Build history of the part. All positions in model axes, mm. Round coordinates to 2 decimals unless told otherwise and drop trailing zeros. Order: outer loops, then holes, each group sorted by start corner. A loop starts at its lowest first (then second) coordinate and runs counter-clockwise, first axis right, second up. Notation, with made-up numbers: (13, -22.75) -> (50, -22.75) arc R25 ccw to (50, -6.75) -> close; hole circle Ø4 at (-33, 29.5). An arc over 180 degrees is marked (long way). Answer as a JSON object with one key per item and string values.
from build123d import *

# Parameters (mm, degrees)
SKETCH_W  = 7
SKETCH_H  = 7
PAD_DEPTH = 60


with BuildPart() as part:
    # Sketch → Pad (new body)
    with BuildSketch(Plane.XY):
        Rectangle(SKETCH_W, SKETCH_H)
        with BuildLine():
            ThreePointArc((-1.349854, 1.608693), (0, -2.1), (1.349854, 1.608693))
            Line((0.764337, 2.1), (1.349854, 1.608693))
            Line((-0.764337, 2.1), (0.764337, 2.1))
            Line((-0.764337, 2.1), (-1.349854, 1.608693))
        make_face(mode=Mode.SUBTRACT)
    extrude(amount=PAD_DEPTH)


solid = part.part
1) Cut at A-A, the plane y = 0. Give the cut face in (x, z), plus the area to 3 significant figures.
Checked values:
{"outline": "(-3.5, 0) -> (-2.1, 0) -> (-2.1, 60) -> (-3.5, 60) -> close; (2.1, 0) -> (3.5, 0) -> (3.5, 60) -> (2.1, 60) -> close", "area": "168 mm²"}
2) Probe L1, parallel to Y at x = 0, z = 25; L2, parallel to Y at x = 1.25, z = 57. List the from-to ranges inside material, lowest first. Write a range as from..to.
Checked values:
{"L1": "y = -3.5..-2.1, 2.1..3.5", "L2": "y = -3.5..-1.69, 1.69..3.5"}
3) Cut at B-B, the plane z = 24.5. Give the cut face in (x, y), plus the area to 3 significant figures.
Checked values:
{"outline": "(-3.5, -3.5) -> (3.5, -3.5) -> (3.5, 3.5) -> (-3.5, 3.5) -> close; hole (-1.35, 1.61) arc R2.1 ccw (long way) to (1.35, 1.61) -> (0.76, 2.1) -> (-0.76, 2.1) -> close", "area": "35.0 mm²"}
4) Flat gauge pin, fed straight in: pin 1 Ø1 at (x, y) = (1, -0.5) entering from -Z. Where does the tip first touch, or does it go through?
Checked values:
{"pin 1": "passes through"}
5) Pull direction X, two halves, no side cores. Call faces 1 (the face through (0, 2.1, 30)), 2 (the face through (0, 3.5, 30)), 3 (the face through (-3.5, 0, 30)): pulls with the +X half, pulls with the -X half, needs draft (parallel to the pull), parting line crosses it, or undercut.
Checked values:
{"face 1": "undercut", "face 2": "needs draft", "face 3": "pulls with the -X half"}
